Could you check a few things on this model? Use its own coordinates, in mm. A direction names the side the tool comes from. Give positions to 0.01 mm unless a question says otherwise; leave off trailing zeros. Loops run counter-clockwise (first coordinate to the right, second up) from the corner with the lowest first, then second, coordinate; pieces in that order, holes last. Notation, with made-up numbers: (21, -20.75) -> (65, -20.75) arc R14 cw to (65, -3.75) -> close; hole circle Ø4 at (-4.75, 24). An arc over 180 degrees is marked (long way). Write each question's results on one line, items separated by ' | '. Start each with the question number.
Q1. If we section it at A-A, the plane x = 290: List the corners of the cut face in (y, z) for me, plus the area to 3 significant figures.
Q2. Which directions (+Z, -Z, +X, -X, +Y, -Y) give clear straight access to the entire face, cutting with the end or side of a thin tool? Please do faces 5 (the face through (295.515, -407, 5)), 6 (the face through (277.523, -409.892, 4.93)), 7 (the face through (288.515, -414, 5)).
Q3. We'd pull the mould along X, two halves only. Please class faces 1 (the face through (280.19, -411.96, 4.93)), 2 (the face through (277.03, -411.01, 4.93)), 3 (the face through (273.285, -406.116, 4.93)), 4 (the face through (293, -412.214, 5)): released by +X, released by -X, zero draft, split by the parting line, or undercut.
Q4. If I drill on line 1 along Y through (x, z) = (282, 5.5); line 2 along Y through (x, z) = (295, 7.75); line 3 along X through (y, z) = (-420.5, 3.75), over which ranges is the centre line in solid material (lowest first)?
Q5. If we section it at C-C, the plane y = -420: List the corners of the cut face in (x, z) for me.
Q6. If we section it at D-D, the plane x = 299.5: List the corners of the cut face in (y, z) for me.
Q7. Will these pins go through, and if not, where does the flat tip stop? P1, Ø1, axis at x = 289.5, z = 5, coming from the -Y side; P2, Ø0.7, axis at y = -412, z = 4, coming from the -X side; P3, Ø0.6, axis at x = 289, z = 4, coming from the -Y side.
from build123d import *

# Parameters (mm, degrees)
DODANIE_WYCI_GNI_CIE1_DEPTH = 10


with BuildPart() as part:
    # Szkic1 → Dodanie-wyciągnięcie1 (new body)
    with BuildSketch(Plane.XY):
        with BuildLine():
            Line((269.016524324, -406.868519497), (271.654292788, -421.82804783))
            ThreePointArc((271.654292788, -421.82804783), (272.538891868, -423.715939148), (274.253329281, -424.902258464))
            Line((274.253329281, -424.902258464), (295.514699013, -432.462846953))
            Line((295.514699013, -432.462846953), (295.514699013, -425.313881279))
            Line((295.514699013, -425.313881279), (301.514699013, -425.313881279))
            Line((301.514699013, -425.313881279), (301.514699013, -419.313881279))
            Line((301.514699013, -419.313881279), (295.514699013, -419.313881279))
            Line((295.514699013, -419.313881279), (295.514699013, -415.313881279))
            Line((295.514699013, -415.313881279), (291.014699013, -415.313881279))
            Line((291.014699013, -415.313881279), (291.014699013, -416.688881279))
            Line((291.014699013, -416.688881279), (289.014699013, -416.688881279))
            Line((289.014699013, -416.688881279), (289.014699013, -415.313881279))
            Line((289.014699013, -415.313881279), (288.514699013, -415.313881279))
            Line((288.514699013, -415.313881279), (288.514699013, -412.213881279))
            Line((288.514699013, -412.213881279), (289.014699013, -412.213881279))
            Line((289.014699013, -412.213881279), (289.014699013, -410.838881279))
            Line((289.014699013, -410.838881279), (291.014699013, -410.838881279))
            Line((291.014699013, -410.838881279), (291.014699013, -412.213881279))
            Line((291.014699013, -412.213881279), (295.514699013, -412.213881279))
            Line((295.514699013, -412.213881279), (295.514699013, -402.150585233))
            Line((295.514699013, -402.150585233), (280.48065548, -404.801492737))
            Line((280.48065548, -404.801492737), (281.26207228, -409.233127626))
            Line((281.26207228, -409.233127626), (282.61618294, -408.994361382))
            Line((282.61618294, -408.994361382), (282.963479295, -410.963976888))
            Line((282.963479295, -410.963976888), (281.609368635, -411.202743132))
            Line((281.609368635, -411.202743132), (281.696192724, -411.695147008))
            Line((281.696192724, -411.695147008), (278.64328869, -412.233456359))
            Line((278.64328869, -412.233456359), (278.556464601, -411.741052483))
            Line((278.556464601, -411.741052483), (277.20235394, -411.979818727))
            Line((277.20235394, -411.979818727), (276.855057585, -410.010203221))
            Line((276.855057585, -410.010203221), (278.209168245, -409.771436977))
            Line((278.209168245, -409.771436977), (277.435547988, -405.384018473))
            Line((277.435547988, -405.384018473), (269.016524324, -406.868519497))
        make_face()
    extrude(amount=DODANIE_WYCI_GNI_CIE1_DEPTH)


solid = part.part
Final values:
1) outline: (-430.5, 0) -> (-416.69, 0) -> (-416.69, 10) -> (-430.5, 10) -> close; (-410.84, 0) -> (-403.12, 0) -> (-403.12, 10) -> (-410.84, 10) -> close | area: 215 mm²
2) face 5: +Z, -Z, +X, +Y | face 6: +Z, -Z | face 7: +Z, -Z, +X
3) face 1: undercut | face 2: undercut | face 3: released by -X | face 4: zero draft
4) line 1: y = -427.66 to -411.13, -409.1 to -404.53 | line 2: y = -432.28 to -415.31, -412.21 to -402.24 | line 3: x = 271.42 to 301.51
5) outline: (271.33, 0) -> (301.51, 0) -> (301.51, 10) -> (271.33, 10) -> close
6) outline: (-425.31, 0) -> (-419.31, 0) -> (-419.31, 10) -> (-425.31, 10) -> close
7) P1: stops at y = -430.5 | P2: stops at x = 269.86 | P3: stops at y = -430.25
